Design review of the part built by this model. Coordinates are the model's own, in mm. Give positions to 0.01 mm unless a question says otherwise; leave off trailing zeros. Write each loop counter-clockwise with the first axis right and the second up, starting at its lowest first coordinate (ties: lowest second). Pieces come first, ordered by that corner, then holes.
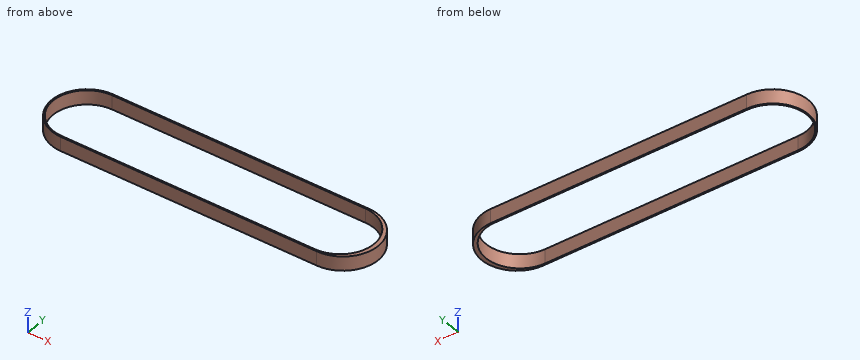
```python
from build123d import *

# Parameters (mm, degrees)
BOSS_EXTRUDE1_DEPTH = 12.7
CUT_EXTRUDE1_DEPTH  = 12.7


with BuildPart() as part:
    # Sketch2 → Boss-Extrude1 (new body)
    with BuildSketch(Plane.XY):
        with BuildLine():
            Line((0, 31.4325), (227.965, 31.4325))
            ThreePointArc((227.965, 31.4325), (259.3975, 0), (227.965, -31.4325))
            Line((227.965, -31.4325), (0, -31.4325))
            ThreePointArc((0, -31.4325), (-31.4325, 0), (0, 31.4325))
        make_face()
    extrude(amount=BOSS_EXTRUDE1_DEPTH)

    # Sketch3 → Cut-Extrude1 (cut)
    with BuildSketch(Plane.XY.offset(12.7)):
        with BuildLine():
            Line((0, 30.1625), (225.425, 30.1625))
            ThreePointArc((225.425, 30.1625), (255.5875, 0), (225.425, -30.1625))
            Line((225.425, -30.1625), (0, -30.1625))
            ThreePointArc((0, -30.1625), (-30.1625, 0), (0, 30.1625))
        make_face()
    extrude(amount=-CUT_EXTRUDE1_DEPTH, mode=Mode.SUBTRACT)


solid = part.part
```
(1) Consider section A-A, the plane y = 0. Give the boundary of the cut face in (x, z), then the cut area to 3 significant figures.
Resolved:
outline: (-31.43, 0) - (-30.16, 0) - (-30.16, 12.7) - (-31.43, 12.7) - close; (255.59, 0) - (259.4, 0) - (259.4, 12.7) - (255.59, 12.7) - close
area: 64.5 mm2
(2) Consider section B-B, the plane z = 10. Give the boundary of the cut face in (x, y) (1 decimal).
Resolved:
outline: (0, -31.4) - (228, -31.4) arc R31.4 ccw to (228, 31.4) - (0, 31.4) arc R31.4 ccw to start; hole (0, -30.2) - (225.4, -30.2) arc R30.2 ccw to (225.4, 30.2) - (0, 30.2) arc R30.2 ccw to start
(3) Clearance check with flat-ended pins moving along their axes: P1, Ø4, axis at y = -15.5, z = 6, coming from the -X side; P2, Ø6, axis at y = -23, z = 2.5, coming from the +X side; P3, Ø1.5, axis at y = -17, z = 6.5, coming from the -X side. State where each tip first meets the part, or that it passes through.
Resolved:
P1: stops at x = -28.39
P2: stops at x = 252.21
P3: stops at x = -26.91
(4) Consider section C-C, the plane x = 22.5. Give the boundary of the cut face in (y, z), then the cut area to 3 significant figures.
Resolved:
outline: (-31.43, 0) - (-30.16, 0) - (-30.16, 12.7) - (-31.43, 12.7) - close; (30.16, 0) - (31.43, 0) - (31.43, 12.7) - (30.16, 12.7) - close
area: 32.3 mm2
(5) To check wall thickness, follow L1, parallel to Y at x = 73.5, z = 7.5; L2, parallel to X at y = 1.5, z = 11; L3, parallel to X at y = 0, z = 9.25. State the ranges of each line that lie inside material, in increasing order.
Resolved:
L1: y = -31.43 to -30.16, 30.16 to 31.43
L2: x = -31.4 to -30.13, 255.55 to 259.36
L3: x = -31.43 to -30.16, 255.59 to 259.4
